```python
from build123d import *

# Parameters (mm, degrees)
F0_R     = 19.05
F1_DEPTH = 101.6
F2_SIZE  = 5.08
F3_R     = 5.08


with BuildPart() as f1:
    # F0 (on Top) → F1 (new body)
    with BuildSketch(Plane.XY):
        Circle(F0_R)
    extrude(amount=F1_DEPTH)

    # F2
    f2_edges = [f1.edges().sort_by_distance(p)[0] for p in [
        (-19.05, 0, 101.6),
        (-19.05, 0, 0),
    ]]
    chamfer(f2_edges, length=F2_SIZE)

    # F3
    f3_edges = [f1.edges().sort_by_distance(p)[0] for p in [
        (19.05, 0, 50.8),
        (-19.05, 0, 5.08),
        (-19.05, 0, 96.52),
        (-13.97, 0, 0),
        (-13.97, 0, 101.6),
    ]]
    fillet(f3_edges, radius=F3_R)


solid = f1.part
```
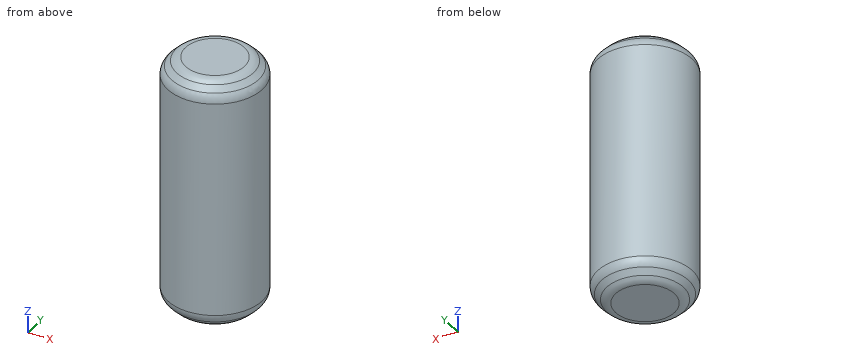
Source: CAD feature listing. Evaluate the final solid. Frame: model axes, mm. Coordinates: 2 decimals unless noted, no trailing zeros. Loops run counter-clockwise (first coordinate to the right, second up) from the corner with the lowest first, then second, coordinate; pieces in that order, holes last. Notation, with made-up numbers: (50, -13.75) - (84, -13.75) arc R32 ccw to (84, 18.25) - close; hole circle Ø2 at (22.25, 1). An arc over 180 degrees is marked (long way). Answer as CSV lines item,"result".
1. Section A-A (z = 10). Return loops of the section in (x, y), then the cut area to 3 significant figures.
Established:
outline,"circle Ø38.1 at (0, 0)"
area,"1,140 mm2"
2. Contact query for flat-ended pins moving along their axis: pin 1 (1.5 mm diameter, centred on y = 12.5, z = 52.5, fed in from -X); pin 2 (3 mm diameter, centred on x = -9.5, y = 9, fed in from -Z); pin 3 (3 mm diameter, centred on y = 9.5, z = 11.5, fed in from -X); pin 4 (8 mm diameter, centred on x = -14.5, z = 34, fed in from -Y). Output: stop coordinate, or through.
Established:
pin 1,"stops at x = -14.99"
pin 2,"stops at z = 0"
pin 3,"stops at x = -17.29"
pin 4,"stops at y = -15.9"
3. Ray query, line 1 (X direction, y = 0, z = 77.5); line 2 (Z direction, x = 5, y = -11); line 3 (Y direction, x = -12, z = 11). Return the intervals inside material, ascending.
Established:
line 1,"x = -19.05 to 19.05"
line 2,"z = 0 to 101.6"
line 3,"y = -14.8 to 14.8"
